from build123d import *

# Parameters (mm, degrees)
F0_W     = 25.4
F0_H     = 25.4
F1_DEPTH = 25.4
F2_R     = 5.08
F3_SIZE  = 5.08
F4_W     = 25.741957128
F4_H     = 25.5791675299
F4_W_2   = 21.6466449201
F4_H_2   = 21.9391710125
F5_DEPTH = 2.54
F6_R     = 1.26999


# Not quite as in the source:
# - a fillet or chamfer is up to 0.001 mm smaller than in the source, because OpenCascade refuses the exact size


with BuildPart() as f1:
    # F0 (on Front) → F1 (new body)
    with BuildSketch(Plane.XZ):
        with Locations((-48.8445848724, -0.7304809988)):
            Rectangle(F0_W, F0_H)
    extrude(amount=F1_DEPTH)

    # F2
    f2_edges = [f1.edges().sort_by_distance(p)[0] for p in [
        (-48.844585, -25.4, 11.969519),
        (-36.144585, -12.7, 11.969519),
        (-48.844585, 0, 11.969519),
        (-61.544585, -12.7, 11.969519),
    ]]
    fillet(f2_edges, radius=F2_R)

    # F3
    f3_edges = [f1.edges().sort_by_distance(p)[0] for p in [
        (-48.844585, -25.4, -13.430481),
        (-36.144585, -12.7, -13.430481),
        (-61.544585, -12.7, -13.430481),
        (-48.844585, 0, -13.430481),
    ]]
    chamfer(f3_edges, length=F3_SIZE)

    # F4 (on Top) → F5 (cut)
    with BuildSketch(Plane.XY):
        with Locations((-48.707395792, -12.789583765)):
            Rectangle(F4_W, F4_H)
        with Locations((-48.4148729593, -12.8544487525)):
            Rectangle(F4_W_2, F4_H_2, mode=Mode.SUBTRACT)
    extrude(amount=-F5_DEPTH, mode=Mode.SUBTRACT)

    # F6 (radius 1.27 in the source; OpenCascade refuses exactly that, so slightly less here)
    f6_edges = [f1.edges().sort_by_distance(p)[0] for p in [
        (-48.414873, -1.884863, -2.54),
        (-37.59155, -12.854449, -2.54),
        (-48.414873, -1.884863, 0),
        (-37.59155, -12.854449, 0),
        (-48.414873, -23.824034, -2.54),
        (-59.238195, -12.854449, -2.54),
        (-48.414873, -23.824034, 0),
        (-59.238195, -12.854449, 0),
    ]]
    fillet(f6_edges, radius=F6_R)


solid = f1.part
Model file for the job. Use its own axes, mm. A direction names the side the tool comes from. Give positions to 0.01 mm unless a question says otherwise; leave off trailing zeros. One line per item, written item: value.
Item 1: Two-plate mould, pull along Z, no slides. Class faces 4 (the flat face through (-36.145, -13, -5)), 5 (the flat face through (-38.649, -12.522, -10.855)), 6 (the cylindrical face through (-48.25, -24.21, -2.18)): released by +Z, released by -Z, zero draft, split by the parting line, or undercut.
Response values:
face 4: zero draft
face 5: released by -Z
face 6: undercut
Item 2: Pin check, flat tips, straight feed: pin 1 Ø2 at (x, y) = (-53, -2.5) entering from +Z; pin 2 Ø1.5 at (x, z) = (-40, -11) entering from +Y; pin 3 Ø2 at (x, y) = (-57.5, -22) entering from -Z. Stop position of each tip, or through.
Response values:
pin 1: z = 11.72
pin 2: y = -1.9
pin 3: z = -12.7
Item 3: Wall check: line 1 (Z direction, x = -60.5, y = -24); line 2 (X direction, y = -21.25, z = -11.75); line 3 (Z direction, x = -49, y = -2.5). Give the ranges that are in metal, low to high.
Response values:
line 1: -9.4 to -2.54, 0 to 9.98
line 2: -58.15 to -39.54
line 3: -10.85 to 11.27
Item 4: Tool access for faces 1 (the flat face through (-49, -25.4, -5)), 2 (the cylindrical face through (-37.21, -12.68, -2.18)), 3 (the cylindrical face through (-59.6, -12.68, -0.38)): list every direction of +Z, -Z, +X, -X, +Y, -Y with a clear straight run to the whole face (end or side of a thin tool).
Response values:
face 1: +Z, -Z, +X, -X, -Y
face 2: +X, +Y, -Y
face 3: -X, +Y, -Y
